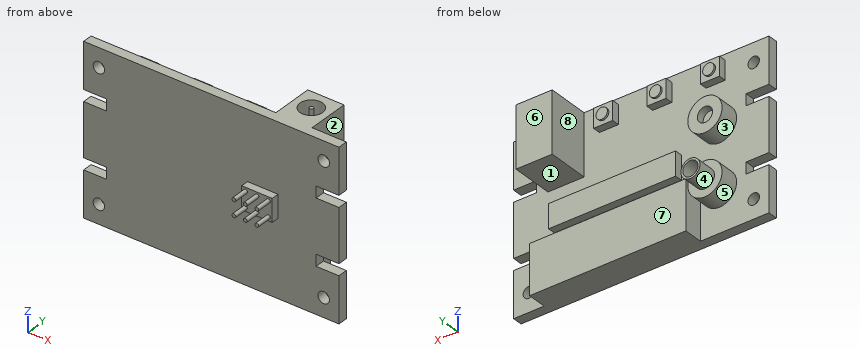
from build123d import *

# Parameters (mm, degrees)
BOSS_EXTRUDE1_DEPTH  = 2.54
SKETCH2_R            = 1.5
CUT_EXTRUDE1_DEPTH   = 3.54
SKETCH3_R            = 4.5
BOSS_EXTRUDE2_DEPTH  = 5
SKETCH4_R            = 2.5
SKETCH4_R_2          = 2
BOSS_EXTRUDE3_DEPTH  = 5
SKETCH5_R            = 2
CUT_EXTRUDE2_DEPTH   = 2
SKETCH6_W            = 41
SKETCH6_H            = 13
BOSS_EXTRUDE4_DEPTH  = 5
SKETCH7_W            = 5
SKETCH7_H            = 5
BOSS_EXTRUDE5_DEPTH  = 2
SKETCH8_R            = 1.5
BOSS_EXTRUDE6_DEPTH  = 0.5
SKETCH9_W            = 9.5
SKETCH9_H            = 16
BOSS_EXTRUDE7_DEPTH  = 11
SKETCH10_R           = 3
SKETCH10_R_2         = 0.5
CUT_EXTRUDE3_DEPTH   = 10
SKETCH11_W           = 33.328489161
SKETCH11_H           = 6.282155695
BOSS_EXTRUDE8_DEPTH  = 2
SKETCH12_W           = 8
SKETCH12_H           = 6
BOSS_EXTRUDE9_DEPTH  = 2
SKETCH13_R           = 0.5
BOSS_EXTRUDE10_DEPTH = 4


with BuildPart() as part:
    # Sketch1 → Boss-Extrude1 (new body)
    with BuildSketch(Plane(origin=(0, 0, 0), x_dir=(1, 0, 0), z_dir=(0, 1, 0))):
        Polygon((-33.5, 10), (-33.5, 22), (33.5, 22), (33.5, 10), (27.5, 10), (27.5, 7), (33.5, 7), (33.5, -7), (27.5, -7), (27.5, -10), (33.5, -10), (33.5, -22), (-33.5, -22), (-33.5, -10), (-27.5, -10), (-27.5, -7), (-33.5, -7), (-33.5, 7), (-27.5, 7), (-27.5, 10), align=None)
    extrude(amount=BOSS_EXTRUDE1_DEPTH)

    # Sketch2 → Cut-Extrude1 (cut, through all)
    with BuildSketch(Plane(origin=(0, 2.54, 0), x_dir=(1, 0, 0), z_dir=(0, 1, 0))):
        with Locations((-29.5, -17)):
            Circle(SKETCH2_R)
        with Locations((-29.5, 17)):
            Circle(SKETCH2_R)
        with Locations((29.5, 17)):
            Circle(SKETCH2_R)
        with Locations((29.5, -17)):
            Circle(SKETCH2_R)
    extrude(amount=-CUT_EXTRUDE1_DEPTH, mode=Mode.SUBTRACT)

    # Sketch3 → Boss-Extrude2 (add)
    with BuildSketch(Plane(origin=(0, 2.54, 0), x_dir=(1, 0, 0), z_dir=(0, 1, 0))):
        with Locations((-20.5, 11)):
            Circle(SKETCH3_R)
        with Locations((-20.5, -5)):
            Circle(SKETCH3_R)
    extrude(amount=BOSS_EXTRUDE2_DEPTH)

    # Sketch4 → Boss-Extrude3 (add)
    with BuildSketch(Plane(origin=(0, 7.54, 0), x_dir=(1, 0, 0), z_dir=(0, 1, 0))):
        with Locations((-20.5, 11)):
            Circle(SKETCH4_R)
        with Locations((-20.5, 11)):
            Circle(SKETCH4_R_2, mode=Mode.SUBTRACT)
    extrude(amount=BOSS_EXTRUDE3_DEPTH)

    # Sketch5 → Cut-Extrude2 (cut)
    with BuildSketch(Plane(origin=(0, 7.54, 0), x_dir=(1, 0, 0), z_dir=(0, 1, 0))):
        with Locations((-20.5, -5)):
            Circle(SKETCH5_R)
    extrude(amount=-CUT_EXTRUDE2_DEPTH, mode=Mode.SUBTRACT)

    # Sketch6 → Boss-Extrude4 (add)
    with BuildSketch(Plane(origin=(0, 2.54, 0), x_dir=(1, 0, 0), z_dir=(0, 1, 0))):
        with Locations((5, 15.5)):
            Rectangle(SKETCH6_W, SKETCH6_H)
    extrude(amount=BOSS_EXTRUDE4_DEPTH)

    # Sketch7 → Boss-Extrude5 (add)
    with BuildSketch(Plane(origin=(0, 2.54, 0), x_dir=(1, 0, 0), z_dir=(0, 1, 0))):
        with Locations((-19.5, -18)):
            Rectangle(SKETCH7_W, SKETCH7_H)
        with Locations((-5.5, -18)):
            Rectangle(SKETCH7_W, SKETCH7_H)
        with Locations((8.5, -18)):
            Rectangle(SKETCH7_W, SKETCH7_H)
    extrude(amount=BOSS_EXTRUDE5_DEPTH)

    # Sketch8 → Boss-Extrude6 (add)
    with BuildSketch(Plane(origin=(0, 4.54, 0), x_dir=(1, 0, 0), z_dir=(0, 1, 0))):
        with Locations((-19.5, -18)):
            Circle(SKETCH8_R)
        with Locations((-5.5, -18)):
            Circle(SKETCH8_R)
        with Locations((8.5, -18)):
            Circle(SKETCH8_R)
    extrude(amount=BOSS_EXTRUDE6_DEPTH)

    # Sketch9 → Boss-Extrude7 (add)
    with BuildSketch(Plane(origin=(0, 2.54, 0), x_dir=(1, 0, 0), z_dir=(0, 1, 0))):
        with Locations((19.75, -14)):
            Rectangle(SKETCH9_W, SKETCH9_H)
    extrude(amount=BOSS_EXTRUDE7_DEPTH)

    # Sketch10 → Cut-Extrude3 (cut)
    with BuildSketch(Plane.XY.offset(22)):
        with Locations((19.75, 8.54)):
            Circle(SKETCH10_R)
        with Locations((19.75, 8.54)):
            Circle(SKETCH10_R_2, mode=Mode.SUBTRACT)
    extrude(amount=-CUT_EXTRUDE3_DEPTH, mode=Mode.SUBTRACT)

    # Sketch11 → Boss-Extrude8 (add)
    with BuildSketch(Plane(origin=(0, 2.54, 0), x_dir=(1, 0, 0), z_dir=(0, 1, 0))):
        with Locations((6.149899785, 1.719326822)):
            Rectangle(SKETCH11_W, SKETCH11_H)
    extrude(amount=BOSS_EXTRUDE8_DEPTH)

    # Sketch12 → Boss-Extrude9 (add)
    with BuildSketch(Plane.XZ):
        with Locations((13.5, 1)):
            Rectangle(SKETCH12_W, SKETCH12_H)
    extrude(amount=BOSS_EXTRUDE9_DEPTH)

    # Sketch13 → Boss-Extrude10 (add)
    with BuildSketch(Plane.XZ.offset(2)):
        with Locations((10.5, 3)):
            Circle(SKETCH13_R)
        with Locations((13.5, 3)):
            Circle(SKETCH13_R)
        with Locations((16.5, 3)):
            Circle(SKETCH13_R)
        with Locations((16.5, -1)):
            Circle(SKETCH13_R)
        with Locations((13.5, -1)):
            Circle(SKETCH13_R)
        with Locations((10.5, -1)):
            Circle(SKETCH13_R)
    extrude(amount=BOSS_EXTRUDE10_DEPTH)


solid = part.part
Design review of the part built by this model. Coordinates are the model's own, in mm. Face numbers are marked on the shaded views. A direction names the side the tool comes from. Coordinates: 2 decimals unless noted, no trailing zeros. Loops run counter-clockwise (first coordinate to the right, second up) from the corner with the lowest first, then second, coordinate; pieces in that order, holes last. Notation, with made-up numbers: M -34,7.25 L 1,7.25 A27 ccw 1,26.25 Z; hole C -1,-8 d3. An arc over 180 degrees is marked long. Answer as CSV lines item,"result".
Item 1: The part is to be moulded in two halves that separate along X. For the marked faces 1, 2, 3 and 4, say which applies: pulls with the +X half, pulls with the -X half, needs draft (parallel to the pull), parting line crosses it, or undercut.
Answer list:
face 1,"needs draft"
face 2,"pulls with the +X half"
face 3,"undercut"
face 4,"parting line crosses it"
Item 2: For P1, Ø2.5, axis at x = -18.5, z = -9, coming from the +Y side; P2, Ø10.5, axis at x = -5, z = -17.5, coming from the +Y side; P3, Ø1.9, axis at x = 0.5, z = -2, coming from the +Y side; P4, Ø2.5, axis at x = -29.5, z = 17, coming from the +Y side, all flat-tipped, find the tip position at first contact; note any pin that passes through.
Answer list:
P1,"y = 12.54"
P2,"y = 7.54"
P3,"y = 4.54"
P4,"through"
Item 3: Add section B-B on z = -17. State the section outline as (x, y) points, plus the area to 3 significant figures.
Answer list:
outline,"M -33.5,0 L -31,0 L -31,2.54 L -33.5,2.54 Z; M -28,0 L 28,0 L 28,2.54 L 25.5,2.54 L 25.5,7.54 L -15.5,7.54 L -15.5,2.54 L -28,2.54 Z; M 31,0 L 33.5,0 L 33.5,2.54 L 31,2.54 Z"
area,"360 mm²"
Item 4: Add section D-D on x = 8.5. State the section outline as (y, z) points, plus the area to 3 significant figures.
Answer list:
outline,"M 0,-22 L 7.54,-22 L 7.54,-9 L 2.54,-9 L 2.54,-4.86 L 4.54,-4.86 L 4.54,1.42 L 2.54,1.42 L 2.54,15.5 L 4.54,15.5 L 4.54,16.5 L 5.04,16.5 L 5.04,19.5 L 4.54,19.5 L 4.54,20.5 L 2.54,20.5 L 2.54,22 L 0,22 Z"
area,"201 mm²"
Item 5: For probe 1 along Z at (x, y) = (-29.5, 1.1); probe 2 along X at (y, z) = (1.1, 17); probe 3 along Z at (x, y) = (-20.5, 6.4), list the stretches that pass through material, from the lowest coordinate up.
Answer list:
probe 1,"-22 to -18.5, -15.5 to -10, -7 to 7, 10 to 15.5, 18.5 to 22"
probe 2,"-33.5 to -31, -28 to 28, 31 to 33.5"
probe 3,"-15.5 to -6.5, 0.5 to 3, 7 to 9.5"
Item 6: Add section A-A on z = 13. State the section outline as (x, y) points.
Answer list:
outline,"M -33.5,0 L 33.5,0 L 33.5,2.54 L 24.5,2.54 L 24.5,13.54 L 15,13.54 L 15,2.54 L -33.5,2.54 Z; C 19.75,8.54 d1; hole C 19.75,8.54 d6"
Item 7: Add section C-C on y = 10.5. State the section outline as (x, z) points.
Answer list:
outline,"C -20.5,-11 d5; M 15,6 L 24.5,6 L 24.5,22 L 22.02,22 L 22.02,12 L 17.48,12 L 17.48,22 L 15,22 Z; hole C -20.5,-11 d4"
Item 8: Machinability: for the marked faces 5, 6, 7 and 8, which of the approach directions +Z, -Z, +X, -X, +Y, -Y give a long, thin tool a straight path to every point of the face, cutting with its end or side? Answer none if there is none.
Answer list:
face 5,"+Y"
face 6,"+Z, -Z, +X, -X, +Y"
face 7,"-Z, +X, +Y"
face 8,"+Z, +Y"
